```python
from build123d import *

# Parameters (mm, degrees)
SKETCH1_R              = 4.041451884
BOSS_EXTRUDE1_DEPTH    = 1.6
CHAMFER1_SIZE          = 0.6
CUT_EXTRUDE1_START     = -3.2
CUT_EXTRUDE1_OUTLINE_R = 2
CUT_EXTRUDE1_DEPTH     = 3.2
CHAMFER2_SIZE          = 0.3


# Read off the part's stored shape, not the designer's step: Cut-Extrude1
with BuildPart() as part:
    # Sketch1 → Boss-Extrude1 (new, symmetric)
    with BuildSketch(Plane.XY):
        Circle(SKETCH1_R)
    extrude(amount=BOSS_EXTRUDE1_DEPTH, both=True)

    # Chamfer1
    chamfer1_edges = [part.edges().sort_by_distance(p)[0] for p in [
        (-4.041451884, 0, -1.6),
        (-4.041451884, 0, 1.6),
    ]]
    chamfer(chamfer1_edges, length=CHAMFER1_SIZE)

    # Cut-Extrude1 outline → Cut-Extrude1 (cut)
    with BuildSketch(Plane.XY.offset(1.6).offset(CUT_EXTRUDE1_START)):
        with BuildLine():
            ThreePointArc((4.041451884, 0), (3.5, 2.020725942), (2.020725942, 3.5))
            Line((2.020725942, 3.5), (4.041451884, 0))
        make_face()
        with BuildLine():
            Line((-2.020725942, 3.5), (2.020725942, 3.5))
            ThreePointArc((2.020725942, 3.5), (0, 4.041451884), (-2.020725942, 3.5))
        make_face()
        with BuildLine():
            Line((-4.041451884, 0), (-2.020725942, 3.5))
            ThreePointArc((-2.020725942, 3.5), (-3.5, 2.020725942), (-4.041451884, 0))
        make_face()
        with BuildLine():
            ThreePointArc((2.020725942, -3.5), (3.5, -2.020725942), (4.041451884, 0))
            Line((4.041451884, 0), (2.020725942, -3.5))
        make_face()
        with BuildLine():
            Line((-2.020725942, -3.5), (-4.041451884, 0))
            ThreePointArc((-4.041451884, 0), (-3.5, -2.020725942), (-2.020725942, -3.5))
        make_face()
        with BuildLine():
            ThreePointArc((-2.020725942, -3.5), (0, -4.041451884), (2.020725942, -3.5))
            Line((2.020725942, -3.5), (-2.020725942, -3.5))
        make_face()
        Circle(CUT_EXTRUDE1_OUTLINE_R)
    extrude(amount=CUT_EXTRUDE1_DEPTH, mode=Mode.SUBTRACT)

    # Chamfer2
    chamfer2_edges = [part.edges().sort_by_distance(p)[0] for p in [
        (-2, 0, -1.6),
        (-2, 0, 1.6),
    ]]
    chamfer(chamfer2_edges, length=CHAMFER2_SIZE)


solid = part.part
```
The model under review builds one solid part; all positions refer to its coordinate system, in mm. Give positions to 0.01 mm unless a question says otherwise; leave off trailing zeros. Write each loop counter-clockwise with the first axis right and the second up, starting at its lowest first coordinate (ties: lowest second). Pieces come first, ordered by that corner, then holes. Notation, with made-up numbers: (-15.5, 29) - (-7.5, 29) arc R29 ccw to (-7.5, 63) - close; hole circle Ø10 at (75, 52). An arc over 180 degrees is marked (long way). Answer in a Markdown table with one row per item. Add a question column.
1. We need section B-B on z = 0.15. Write out the cut boundary in (x, y).
2. Wall thickness on line 1 along Y through (x, z) = (0, 1.2); line 2 along X through (y, z) = (-1.5, 0.6); line 3 along Y through (x, z) = (-1, 0.65): over which ranges is each line inside the solid? List them lowest first. Write a range as [from, to].
3. We need section D-D on z = -1.15. Write out the cut boundary in (x, y).
4. We need section A-A on x = 0. Write out the cut boundary in (y, z), then the cut area to 3 significant figures.
5. We need section C-C on z = 1.45. Write out the cut boundary in (x, y).
6. Draft analysis for pull direction X (two halves, no side actions). For faces 1 (the cylindrical face through (0, -2, 0)), 2 (the flat face through (3, 1.8, 0)), 3 (the flat face through (-3.045, 1.726, -0.022)), 4 (the flat face through (0, -3.5, 0)), state which applies: +X half, -X half, draft (parallel to the pull), parting line (faces both ways), or undercut.
Ans:
| question | item | result |
|---|---|---|
| 1 | outline | (-4.04, 0) - (-2.02, -3.5) - (2.02, -3.5) - (4.04, 0) - (2.02, 3.5) - (-2.02, 3.5) - close; hole circle Ø4 at (0, 0) |
| 2 | line 1 | y = [-3.5, -2], [2, 3.5] |
| 2 | line 2 | x = [-3.18, -1.32], [1.32, 3.18] |
| 2 | line 3 | y = [-3.5, -1.73], [1.73, 3.5] |
| 3 | outline | (-3.88, -0.28) - (-2.18, -3.22) arc R3.89 ccw to (-1.7, -3.5) - (1.7, -3.5) arc R3.89 ccw to (2.18, -3.22) - (3.88, -0.28) arc R3.89 ccw to (3.88, 0.28) - (2.18, 3.22) arc R3.89 ccw to (1.7, 3.5) - (-1.7, 3.5) arc R3.89 ccw to (-2.18, 3.22) - (-3.88, 0.28) arc R3.89 ccw to start; hole circle Ø4 at (0, 0) |
| 4 | outline | (-3.5, -1.54) - (-3.44, -1.6) - (-2.3, -1.6) - (-2, -1.3) - (-2, 1.3) - (-2.3, 1.6) - (-3.44, 1.6) - (-3.5, 1.54) - close; (2, -1.3) - (2.3, -1.6) - (3.44, -1.6) - (3.5, -1.54) - (3.5, 1.54) - (3.44, 1.6) - (2.3, 1.6) - (2, 1.3) - close |
| 4 | area | 9.41 mm^2 |
| 5 | outline | (-3.43, -1.05) - (-2.63, -2.45) arc R3.59 ccw to (-0.81, -3.5) - (0.81, -3.5) arc R3.59 ccw to (2.63, -2.45) - (3.43, -1.05) arc R3.59 ccw to (3.43, 1.05) - (2.63, 2.45) arc R3.59 ccw to (0.81, 3.5) - (-0.81, 3.5) arc R3.59 ccw to (-2.63, 2.45) - (-3.43, 1.05) arc R3.59 ccw to start; hole circle Ø4.3 at (0, 0) |
| 6 | face 1 | undercut |
| 6 | face 2 | +X half |
| 6 | face 3 | -X half |
| 6 | face 4 | draft |
